```python
from build123d import *

# Parameters (mm, degrees)
BASE_FLANGE3_DEPTH = 35.5
FILLET1_R          = 7.8
CUT_EXTRUDE1_DEPTH = 128.108455757


# Sheet-metal steps are written as plain solids
with BuildPart() as part:
    # Sketch1 → Base-Flange3 (new, symmetric)
    with BuildSketch(Plane(origin=(0, 0, 0), x_dir=(0, 0, -1), z_dir=(1, 0, 0))):
        with BuildLine():
            Line((0, 0), (10.146233816, 0))
            ThreePointArc((10.146233816, 0), (15.312460153, 1.027626311), (19.692175362, 3.954058454))
            Line((19.692175362, 3.954058454), (31.784058454, 16.045941546))
            ThreePointArc((31.784058454, 16.045941546), (36.163773663, 18.972373689), (41.33, 20))
            Line((41.33, 20), (119.83, 20))
            Line((119.83, 20), (119.83, 23.175))
            Line((119.83, 23.175), (41.33, 23.175))
            ThreePointArc((41.33, 23.175), (34.948753765, 21.905691205), (29.538994424, 18.291005576))
            Line((29.538994424, 18.291005576), (17.447111332, 6.199122484))
            ThreePointArc((17.447111332, 6.199122484), (14.097440255, 3.960943827), (10.146233816, 3.175))
            Line((10.146233816, 3.175), (0, 3.175))
            Line((0, 3.175), (0, 0))
        make_face()
    extrude(amount=BASE_FLANGE3_DEPTH, both=True)

    # Fillet1
    fillet1_edges = [part.edges().sort_by_distance(p)[0] for p in [
        (-35.5, 1.5875, 0),
        (-35.5, 21.5875, -119.83),
        (35.5, 1.5875, 0),
        (35.5, 21.5875, -119.83),
    ]]
    fillet(fillet1_edges, radius=FILLET1_R)

    # Sketch15 → Cut-Extrude1 (cut, through all)
    with BuildSketch(Plane(origin=(0, 23.175, 0), x_dir=(1, 0, 0), z_dir=(0, 1, 0))):
        with BuildLine():
            Line((-26.725, 115.83), (26.725, 115.83))
            ThreePointArc((26.725, 115.83), (30.10143488, 114.43143488), (31.5, 111.055))
            Line((31.5, 111.055), (31.5, 8.2))
            ThreePointArc((31.5, 8.2), (30.474873734, 5.725126266), (28, 4.7))
            Line((28, 4.7), (-28, 4.7))
            ThreePointArc((-28, 4.7), (-30.474873734, 5.725126266), (-31.5, 8.2))
            Line((-31.5, 8.2), (-31.5, 111.055))
            ThreePointArc((-31.5, 111.055), (-30.10143488, 114.43143488), (-26.725, 115.83))
        make_face()
    extrude(amount=-CUT_EXTRUDE1_DEPTH, mode=Mode.SUBTRACT)


solid = part.part
```
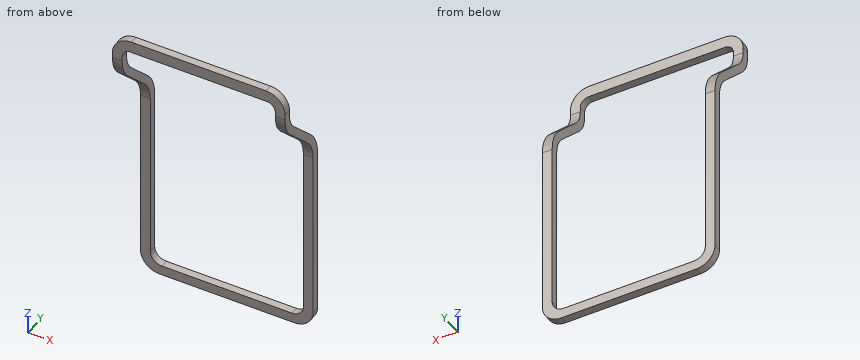
The listing builds one solid part. Answer for the finished solid, in the listing's coordinates (mm). Give positions to 0.01 mm unless a question says otherwise; leave off trailing zeros. Loops run counter-clockwise (first coordinate to the right, second up) from the corner with the lowest first, then second, coordinate; pieces in that order, holes last. Notation, with made-up numbers: (75, 57) - (127, 57) arc R13 cw to (127, 62) - close; hole circle Ø8 at (10, -32.75). An arc over 180 degrees is marked (long way). Answer as CSV lines item,"result". Start each with the question number.
Item 1: Find the intervals of material crossed by line 1 (X direction, y = 21, z = -92); line 2 (Z direction, x = -2, y = 20.5); line 3 (Z direction, x = -18.5, y = 1.5), in increasing order. Write a range as from..to.
Item 2: Each of these flat-tipped pins is pushed along its axis until it touches: pin 1 (1 mm diameter, centred on x = 9, y = 22, fed in from +Z); pin 2 (12 mm diameter, centred on x = -5.5, y = 12.5, fed in from -Z); pin 3 (3 mm diameter, centred on x = -2.5, z = -4, fed in from +Y) (3 decimals); pin 4 (1.6 mm diameter, centred on x = 3, y = 2, fed in from -Z). Where does it stop, or does it pass through?
Item 3: A cutting plane is placed at A-A on z = -59. Determine the outline of the cut face in (x, y) (3 decimals), then the cut area to 3 significant figures.
Item 4: A cutting plane is placed at B-B on x = 21. Determine the outline of the cut face in (y, z) (3 decimals).
Found:
1,line 1,"x = -35.5..-31.5, 31.5..35.5"
1,line 2,"z = -119.83..-115.83"
1,line 3,"z = -4.7..0"
2,pin 1,"stops at z = -115.83"
2,pin 2,"passes through"
2,pin 3,"stops at y = 3.175"
2,pin 4,"stops at z = -4.7"
3,outline,"(-35.5, 20) - (-31.5, 20) - (-31.5, 23.175) - (-35.5, 23.175) - close; (31.5, 20) - (35.5, 20) - (35.5, 23.175) - (31.5, 23.175) - close"
3,area,"25.4 mm^2"
4,outline,"(0, -4.7) - (3.175, -4.7) - (3.175, 0) - (0, 0) - close; (20, -119.83) - (23.175, -119.83) - (23.175, -115.83) - (20, -115.83) - close"
